Autodesk Inventor part; units mm, degrees
ref_plane "YZ Plane" through (0, 0, 0) normal (1, 0, 0) x (0, 1, 0)
ref_plane "XZ Plane" through (0, 0, 0) normal (0, 1, 0) x (-1, 0, 0)
ref_plane "XY Plane" through (0, 0, 0) normal (0, 0, 1) x (1, 0, 0)
sketch "Sketch1" plane through (0, 0, 0) normal (0, 1, 0) x (-1, 0, 0)
  circle A0 centre (0, 0) radius 14
  circle A1 centre (0, 0) radius 15
  dimension "d0" = 1
  dimension "d1" = 28
extrude "Extrusion1" add sketch "Sketch1" along normal blind 15
sketch "Sketch2" plane through (0, 0, 0) normal (0, 0, 1) x (1, 0, 0)
  line L0 (15, 15) -> (-15, 15)
  line L1 (-3.5, 15) -> (3.5, 15)
  line L2 (3.5, 15) -> (3.5, 10)
  line L3 (3.5, 10) -> (-3.5, 10)
  line L4 (-3.5, 10) -> (-3.5, 15)
  point P0 (0, 0)
  point P1 (0, 10)
  dimension "d4" = 7
  dimension "d5" = 5
extrude "Extrusion2" cut sketch "Sketch2" along normal through all both and the other way through all
fillet "Fillet1" radius 0.4 1 edges at (14, 0, 0)
properties part number "tensioner_base"
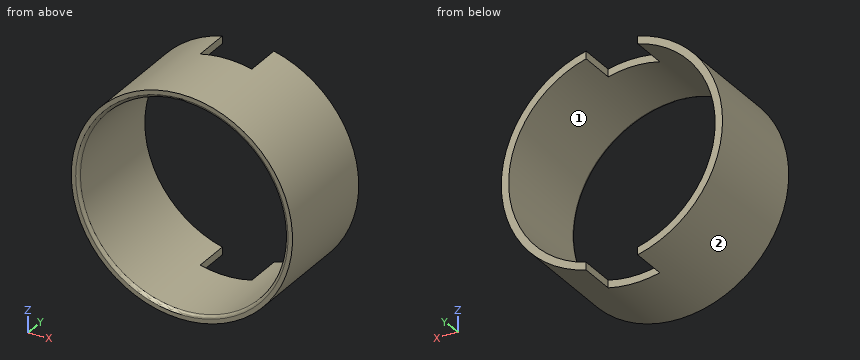
Source: CAD feature listing. Evaluate the final solid. Frame: model axes, mm. Face numbers are marked on the shaded views. Give positions to 0.01 mm unless a question says otherwise; leave off trailing zeros. Loops run counter-clockwise (first coordinate to the right, second up) from the corner with the lowest first, then second, coordinate; pieces in that order, holes last. Notation, with made-up numbers: (15.25, 22.5) -> (73.25, 22.5) arc R4 ccw to (73.25, 26.5) -> close; hole circle Ø11 at (68, 75.25). An arc over 180 degrees is marked (long way). Put each result on its own line as item: value. Start each with the question number.
1) Contact query for flat-ended pins moving along their axis: P1, Ø3, axis at y = 7.5, z = 3.5, coming from the +X side; P2, Ø0.7, axis at x = 0.5, z = -14, coming from the +Y side; P3, Ø1.5, axis at y = 7.5, z = -8, coming from the +X side. Output: stop coordinate, or through.
2) Cut plane A-A (y = 13.75). Return loops of the section in (x, z), then the cut area to 3 significant figures.
3) Material intervals for probe 1 along X at (y, z) = (14, -3.5); probe 2 along Z at (x, y) = (0, 7); probe 3 along X at (y, z) = (1, -6.5), sorted ascending.
4) Cut plane B-B (z = 0). Return loops of the section in (x, y), then the cut area to 3 significant figures.
5) Draft query along Z for the marked faces 1 and 2. Return one class per face: released by +Z, released by -Z, zero draft, split by the parting line, or undercut.
6) Cut plane D-D (y = 2.75). Return loops of the section in (x, z).
7) Cut plane C-C (x = 0). Return loops of the section in (y, z), then the cut area to 3 significant figures.
Results are:
1. P1: stops at x = 14.87
1. P2: stops at y = 10
1. P3: stops at x = 13.13
2. outline: (-3.5, -14.59) -> (-3.5, -13.56) arc R14 cw to (-3.5, 13.56) -> (-3.5, 14.59) arc R15 ccw to start; (3.5, -14.59) arc R15 ccw to (3.5, 14.59) -> (3.5, 13.56) arc R14 cw to (3.5, -13.56) -> close
2. area: 77.0 mm2
3. probe 1: x = -14.59 to -13.56, 13.56 to 14.59
3. probe 2: z = -15 to -14, 14 to 15
3. probe 3: x = -13.52 to -12.4, 12.4 to 13.52
4. outline: (-15, 0) -> (-14.4, 0) arc R0.4 ccw to (-14, 0.4) -> (-14, 15) -> (-15, 15) -> close; (14, 0.4) arc R0.4 ccw to (14.4, 0) -> (15, 0) -> (15, 15) -> (14, 15) -> close
4. area: 29.9 mm2
5. face 1: undercut
5. face 2: split by the parting line
6. outline: circle Ø30 at (0, 0); hole circle Ø28 at (0, 0)
7. outline: (0, -15) -> (10, -15) -> (10, -14) -> (0.4, -14) arc R0.4 ccw to (0, -14.4) -> close; (0, 14.4) arc R0.4 ccw to (0.4, 14) -> (10, 14) -> (10, 15) -> (0, 15) -> close
7. area: 19.9 mm2
